Answer from the drawing. Dimensions are ordinates in mm from the lowest x, y and z of the part. Coordinates: 2 decimals unless noted, no trailing zeros. Order: outer loops, then holes, each group sorted by start corner. A loop starts at its lowest first (then second) coordinate and runs counter-clockwise, first axis right, second up. Notation, with made-up numbers: M -12,30 L -3,30 A18 cw -3,54 Z; hole C 7,18 d6. An arc over 180 degrees is marked long. Use a Markdown table: item, result.
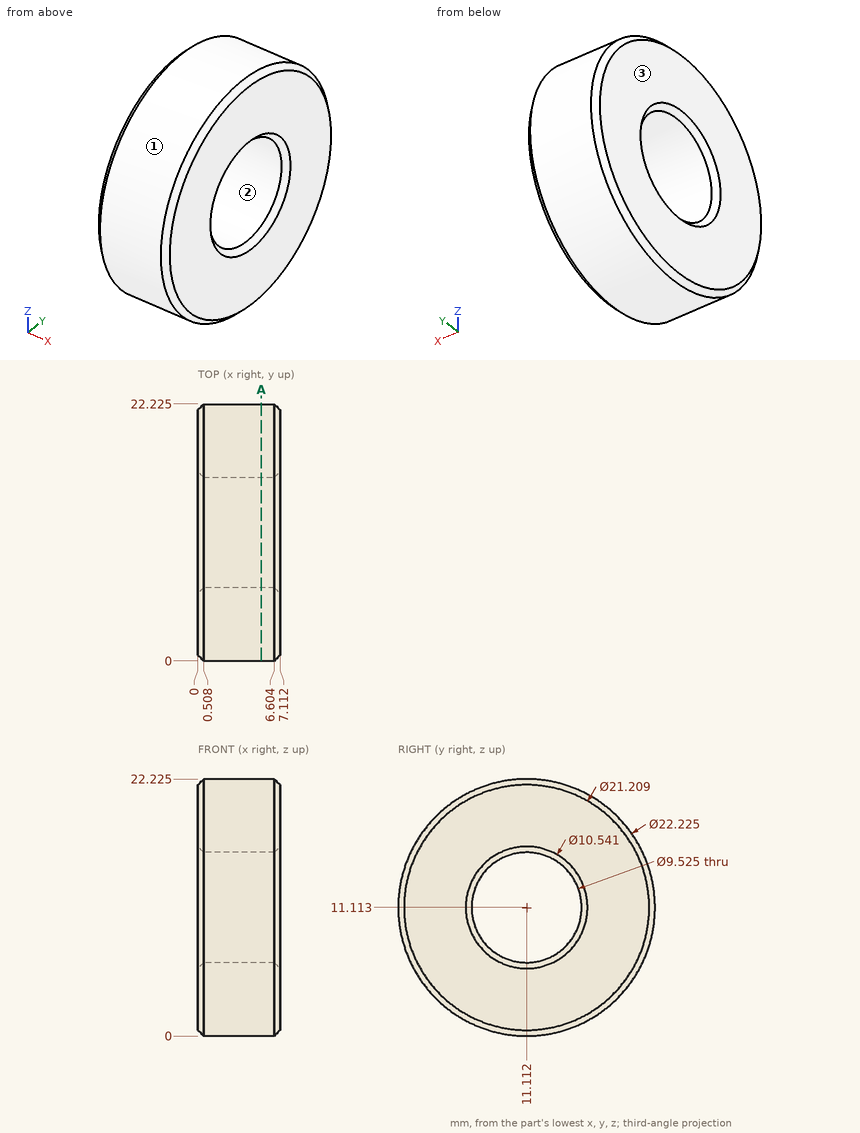
(1) A cutting plane is placed at A-A (x = 5.5). Determine the outline of the cut face in (y, z) (1 decimal), then the cut area to 3 significant figures.
Conclusion:
| item | result |
|---|---|
| outline | C 11.1,11.1 d22.2; hole C 11.1,11.1 d9.5 |
| area | 317 mm2 |
(2) Given P1, Ø3, axis at x = 5.5, z = 3, coming from the +Y side (1 decimal); P2, Ø1.5, axis at x = 2.5, y = 4, coming from the +Z side, each flat-ended and moving along its own axis, determine where each tip first touches the part or whether it passes through.
Conclusion:
| item | result |
|---|---|
| P1 | y = 20 |
| P2 | z = 20.22 |
(3) Determine the mould class of the marked faces 1, 2 and 3 for opening direction Y: pulls with the +Y half, pulls with the -Y half, needs draft (parallel to the pull), parting line crosses it, or undercut.
Conclusion:
| item | result |
|---|---|
| face 1 | parting line crosses it |
| face 2 | undercut |
| face 3 | needs draft |
(4) Straight lines are drawn through the part: L1, parallel to Z at x = 2.5, y = 14.5 (1 decimal); L2, parallel to Z at x = 1.25, y = 10.5 (1 decimal); L3, parallel to Y at x = 2.5, z = 20.5 (1 decimal). For each, find the intervals that lie inside material, in ascending order.
Conclusion:
| item | result |
|---|---|
| L1 | 0.5 to 7.8, 14.5 to 21.7 |
| L2 | 0 to 6.4, 15.8 to 22.2 |
| L3 | 5.2 to 17.1 |
